from build123d import *

# Parameters (mm, degrees)
F0_W     = 25.4
F0_H     = 3.175
F1_DEPTH = 3.175


with BuildPart() as f1:
    # F0 (on Front) → F1 (new body)
    with BuildSketch(Plane.XZ):
        Polygon((-63.5, -38.1), (63.5, -38.1), (63.5, -7.62), (60.325, -7.62), (60.325, -2.0828), (58.42, -2.0828), (58.42, -4.572), (54.9402, -4.572), (54.9402, -2.0828), (50.165, -2.0828), (50.165, 2.0828), (54.9402, 2.0828), (54.9402, 4.572), (58.42, 4.572), (58.42, 2.0828), (60.325, 2.0828), (60.325, 7.62), (63.5, 7.62), (63.5, 38.1), (-63.5, 38.1), align=None)
        with Locations((0, -31.4325)):
            Rectangle(F0_W, F0_H, mode=Mode.SUBTRACT)
    extrude(amount=F1_DEPTH)


solid = f1.part
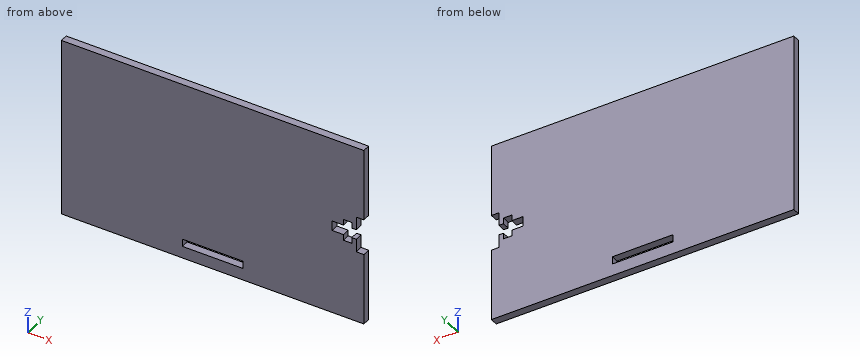
The listing builds one solid part. Answer for the finished solid, in the listing's coordinates (mm). Round coordinates to 2 decimals unless told otherwise and drop trailing zeros. Write each loop counter-clockwise with the first axis right and the second up, starting at its lowest first coordinate (ties: lowest second). Pieces come first, ordered by that corner, then holes. Notation, with made-up numbers: M 67,80 L 116,80 A29 ccw 116,102 Z; hole C 53.25,16.5 d4. An arc over 180 degrees is marked long. Write each question's results on one line, items separated by ' | '. Start each with the question number.
Item 1: Straight lines are drawn through the part: probe 1 along Z at (x, y) = (57, -2.9); probe 2 along X at (y, z) = (-1.1, -31.5); probe 3 along X at (y, z) = (-0.65, 4) (3 decimals). For each, find the intervals that lie inside material, in ascending order.
Item 2: Find section A-A on x = 0. Write down the section's boundary in (y, z) (3 decimals).
Item 3: Find section B-B on y = -1.85. Write down the section's boundary in (x, z) (3 decimals), and give its area (3 significant figures).
Item 4: Given pin 1 Ø1.6 at (y, z) = (-2.5, 5.5) entering from +X (3 decimals), flat-ended and moving along its own axis, determine where the tip first touches the part or whether it passes through.
Answer block:
1) probe 1: z = -38.1 to -4.57, 4.57 to 38.1 | probe 2: x = -63.5 to -12.7, 12.7 to 63.5 | probe 3: x = -63.5 to 54.94, 58.42 to 60.325
2) outline: M -3.175,-38.1 L 0,-38.1 L 0,-33.02 L -3.175,-33.02 Z; M -3.175,-29.845 L 0,-29.845 L 0,38.1 L -3.175,38.1 Z
3) outline: M -63.5,-38.1 L 63.5,-38.1 L 63.5,-7.62 L 60.325,-7.62 L 60.325,-2.083 L 58.42,-2.083 L 58.42,-4.572 L 54.94,-4.572 L 54.94,-2.083 L 50.165,-2.083 L 50.165,2.083 L 54.94,2.083 L 54.94,4.572 L 58.42,4.572 L 58.42,2.083 L 60.325,2.083 L 60.325,7.62 L 63.5,7.62 L 63.5,38.1 L -63.5,38.1 Z; hole M -12.7,-33.02 L 12.7,-33.02 L 12.7,-29.845 L -12.7,-29.845 Z | area: 9,490 mm²
4) pin 1: stops at x = 60.325
